Source: CAD feature listing. Evaluate the final solid. Frame: model axes, mm. A direction names the side the tool comes from. Give positions to 0.01 mm unless a question says otherwise; leave off trailing zeros. Order: outer loops, then holes, each group sorted by start corner. A loop starts at its lowest first (then second) coordinate and runs counter-clockwise, first axis right, second up.
from build123d import *

# Parameters (mm, degrees)
F0_R      = 1.5
F1_DEPTH  = 3
F3_DEPTH  = 18
F2_W      = 10
F2_H      = 7.5
F4_DEPTH  = 20
F5_R      = 3.5
F6_DEPTH  = 3
F7_R      = 2.75
F8_DEPTH  = 25
F9_R      = 1
F10_DEPTH = 25
F11_R     = 3.5
F12_DEPTH = 3


with BuildPart() as f1:
    # F0 (on Top) → F1 (new body)
    with BuildSketch(Plane.XY):
        Polygon((0, 55), (0, 0), (35, 0), (35, 24), (15.932095, 55), align=None)
        with Locations((14, 4)):
            Circle(F0_R, mode=Mode.SUBTRACT)
        with Locations((31, 4)):
            Circle(F0_R, mode=Mode.SUBTRACT)
        with Locations((14, 50)):
            Circle(F0_R, mode=Mode.SUBTRACT)
        Polygon((15.932095, 24), (15.932095, 43.857069), (28.146053, 24), align=None, mode=Mode.SUBTRACT)
    extrude(amount=F1_DEPTH)

    # F2 (on face) → F3 (join)
    with BuildSketch(Plane.XY.offset(3)):
        Polygon((28, 9), (35, 9), (35, 24), (28.146053, 24), (28, 24), align=None)
    extrude(amount=F3_DEPTH)

    # F2 (on face) → F4 (join)
    with BuildSketch(Plane.XY.offset(3)):
        with Locations((5, 3.75)):
            Rectangle(F2_W, F2_H)
        with Locations((5, 51.25)):
            Rectangle(F2_W, F2_H)
    extrude(amount=F4_DEPTH)

    # F5 (on face) → F6 (cut)
    with BuildSketch(Plane(origin=(28, 0, 0), x_dir=(0, -1, 0), z_dir=(-1, 0, 0))):
        with Locations((-16.5, 13)):
            Circle(F5_R)
    extrude(amount=-F6_DEPTH, mode=Mode.SUBTRACT)

    # F7 (on face) → F8 (cut)
    with BuildSketch(Plane(origin=(31, 0, 0), x_dir=(0, -1, 0), z_dir=(-1, 0, 0))):
        with Locations((-16.5, 13)):
            Circle(F7_R)
    extrude(amount=-F8_DEPTH, mode=Mode.SUBTRACT)

    # F9 (on face) → F10 (cut)
    with BuildSketch(Plane(origin=(0, 0, 0), x_dir=(0, -1, 0), z_dir=(-1, 0, 0))):
        with Locations((-2.5, 18)):
            Circle(F9_R)
        with Locations((-2.5, 8)):
            Circle(F9_R)
        with Locations((-52.5, 18)):
            Circle(F9_R)
        with Locations((-52.5, 8)):
            Circle(F9_R)
    extrude(amount=-F10_DEPTH, mode=Mode.SUBTRACT)

    # F11 (on face) → F12 (cut)
    with BuildSketch(Plane.YZ.offset(35)):
        with Locations((16.5, 13)):
            Circle(F11_R)
    extrude(amount=-F12_DEPTH, mode=Mode.SUBTRACT)


solid = f1.part
(1) Line query: line 1 along Y through (x, z) = (14, 1.2); line 2 along Z through (x, y) = (6, 2); line 3 along Z through (x, y) = (28.6, 16.5). Output: solid intervals per line, ascending.
(2) Access query for faces 1 (the flat face through (31, 9, 12)), 2 (the flat face through (15.932, 34, 1)), 3 (the flat face through (13, 28, 3)), 4 (the flat face through (10, 4, 13)). Directions: +Z, -Z, +X, -X, +Y, -Y. A direction counts if a zero-diameter tool reaches every point of the face in a straight line with its end or side. Return the directions, or none.
(3) Section D-D, the plane z = 14.25. Return loops of the section in (x, y).
(4) Pin query (flat end, axial travel): pin 1 Ø6 at (x, z) = (24, 15) entering from +Y; pin 2 Ø10 at (x, z) = (25.5, 13) entering from -Y; pin 3 Ø9.5 at (x, z) = (25.5, 15.5) entering from +Y; pin 4 Ø7.5 at (x, y) = (33, 19) entering from +Z. Return the tip coordinate at first contact, or that it passes through.
(5) Section C-C, the plane z = 18. Return loops of the section in (x, y), plus the area to 3 significant figures.
(6) Draft query along Y for faces 5 (the flat face through (25.6, 39.28, 1.48)), 6 (the cylindrical face through (4.93, 52.63, 8.99)), 7 (the flat face through (31, 17, 21)), 8 (the flat face through (5, 7.5, 13)). Return one class per face: +Y half, -Y half, draft (parallel to the pull), parting line (faces both ways), or undercut.
(7) Section B-B, the plane y = 16.5. Return loops of the section in (x, z), plus the area to 4 significant figures.
(8) Section A-A, the plane z = 5.5. Return loops of the section in (x, y).
Checks:
1. line 1: y = 0 to 2.5, 5.5 to 48.5, 51.5 to 55
1. line 2: z = 0 to 7.13, 8.87 to 17.13, 18.87 to 23
1. line 3: z = 0 to 9.5, 16.5 to 21
2. face 1: +Z, +X, -X, -Y
2. face 2: +Z, -Z
2. face 3: +Z
2. face 4: +Z, +X, +Y, -Y
3. outline: (0, 0) - (10, 0) - (10, 7.5) - (0, 7.5) - close; (0, 47.5) - (10, 47.5) - (10, 55) - (0, 55) - close; (28, 9) - (35, 9) - (35, 13.23) - (32, 13.23) - (32, 14.05) - (31, 14.05) - (31, 13.23) - (28, 13.23) - close; (28, 19.77) - (31, 19.77) - (31, 18.95) - (32, 18.95) - (32, 19.77) - (35, 19.77) - (35, 24) - (28, 24) - close
4. pin 1: passes through
4. pin 2: stops at y = 9
4. pin 3: stops at y = 24
4. pin 4: stops at z = 21
5. outline: (0, 0) - (10, 0) - (10, 1.5) - (0, 1.5) - close; (0, 3.5) - (10, 3.5) - (10, 7.5) - (0, 7.5) - close; (0, 47.5) - (10, 47.5) - (10, 51.5) - (0, 51.5) - close; (0, 53.5) - (10, 53.5) - (10, 55) - (0, 55) - close; (28, 9) - (35, 9) - (35, 24) - (28, 24) - close
5. area: 215 mm2
6. face 5: +Y half
6. face 6: undercut
6. face 7: draft
6. face 8: undercut
7. outline: (0, 0) - (35, 0) - (35, 9.5) - (32, 9.5) - (32, 10.25) - (31, 10.25) - (31, 9.5) - (28, 9.5) - (28, 3) - (0, 3) - close; (28, 16.5) - (31, 16.5) - (31, 15.75) - (32, 15.75) - (32, 16.5) - (35, 16.5) - (35, 21) - (28, 21) - close
7. area: 183.5 mm2
8. outline: (0, 0) - (10, 0) - (10, 7.5) - (0, 7.5) - close; (0, 47.5) - (10, 47.5) - (10, 55) - (0, 55) - close; (28, 9) - (35, 9) - (35, 24) - (28, 24) - close
